Model file for the job. Use its own axes, mm. A direction names the side the tool comes from. Round coordinates to 2 decimals unless told otherwise and drop trailing zeros. Loops run counter-clockwise (first coordinate to the right, second up) from the corner with the lowest first, then second, coordinate; pieces in that order, holes last.
from build123d import *

# Parameters (mm, degrees)
SKETCH_1_R          = 1.5
EXTRUDE_1_DEPTH     = 25
SKETCH_2_R          = 2
SKETCH_2_W          = 5
SKETCH_2_H          = 10
CUT_EXTRUDE_1_DEPTH = 7.5
CHAMFER_1_SIZE      = 1


with BuildPart() as part:
    # 草图1 → 凸台-拉伸1 (new body)
    with BuildSketch(Plane.XY):
        with BuildLine():
            Line((0, -2.5), (-13.5, -2.5))
            Line((-13.5, -2.5), (-13.5, -1.5))
            Line((-13.5, -1.5), (-2, -1.5))
            ThreePointArc((-2, -1.5), (1.118033989, 2.236067977), (0, -2.5))
        make_face()
        Circle(SKETCH_1_R, mode=Mode.SUBTRACT)
    extrude(amount=EXTRUDE_1_DEPTH)

    # 草图2 → 切除-拉伸1 (cut, symmetric)
    with BuildSketch(Plane(origin=(0, -1.5, 0), x_dir=(1, 0, 0), z_dir=(0, 1, 0))):
        with Locations(Location((-9.25, -5, 0), (0, 0, 180))):
            Circle(SKETCH_2_R)
        with Locations(Location((-9.25, -20, 0), (0, 0, 180))):
            Circle(SKETCH_2_R)
        with Locations((0, -12.5)):
            Rectangle(SKETCH_2_W, SKETCH_2_H)
    extrude(amount=CUT_EXTRUDE_1_DEPTH, both=True, mode=Mode.SUBTRACT)

    # 倒角1
    chamfer_1_edges = [part.edges().sort_by_distance(p)[0] for p in [
        (-7.25, -1.5, 5),
        (-7.25, -1.5, 20),
    ]]
    chamfer(chamfer_1_edges, length=CHAMFER_1_SIZE - 0.0001)  # a hair under: the kernel refuses the full size


solid = part.part
Q1. Slice it at B-B on y = 0. Give the cut face in (x, z).
Q2. Flat gauge pins, fed straight in: P1, Ø3.5, axis at x = -5, z = 7.5, coming from the +Y side; P2, Ø4.5, axis at x = -9.25, z = 20, coming from the +Y side; P3, Ø0.8, axis at y = -2, z = 13.5, coming from the +X side. Where does each tip first touch, or does it go through?
Q3. Slice it at D-D on y = 2. Give the cut face in (x, z).
Q4. Probe line 1 (X direction, y = 0, z = 5); line 2 (Z direction, x = -1.75, y = 1.15). List the from-to ranges inside material, lowest first.
Q5. Slice it at A-A on z = 20. State how many separate pieces and enclosed holes the cut face has, plus the area to 3 significant figures.
Q6. Tool access for faces 4 (the face through (-13.5, -2, 12)), 5 (the face through (0, -2, 7.5)): list every direction of +Z, -Z, +X, -X, +Y, -Y with a clear straight run to the whole face (end or side of a thin tool).
Q7. Pull direction Z, two halves, no side cores. Call faces 1 (the face through (-4, -2, 0)), 2 (the face through (0, -2, 17.5)), 3 (the face through (-1.5, 0.07, 21.2)): pulls with the +Z half, pulls with the -Z half, needs draft (parallel to the pull), parting line crosses it, or undercut.
Reply:
1. outline: (-2.5, 0) - (-1.5, 0) - (-1.5, 7.5) - (-2.5, 7.5) - close; (-2.5, 17.5) - (-1.5, 17.5) - (-1.5, 25) - (-2.5, 25) - close; (1.5, 0) - (2.5, 0) - (2.5, 7.5) - (1.5, 7.5) - close; (1.5, 17.5) - (2.5, 17.5) - (2.5, 25) - (1.5, 25) - close
2. P1: stops at y = -1.5
2. P2: stops at y = -2.25
2. P3: stops at x = -2.5
3. outline: (-1.5, 0) - (1.5, 0) - (1.5, 7.5) - (-1.5, 7.5) - close; (-1.5, 17.5) - (1.5, 17.5) - (1.5, 25) - (-1.5, 25) - close
4. line 1: x = -2.5 to -1.5, 1.5 to 2.5
4. line 2: z = 0 to 7.5, 17.5 to 25
5. separate pieces: 2
5. enclosed holes: 1
5. area: 19.7 mm2
6. face 4: +Z, -Z, -X, +Y, -Y
6. face 5: +X, +Y, -Y
7. face 1: pulls with the -Z half
7. face 2: undercut
7. face 3: needs draft
